```python
from build123d import *

# Parameters (mm, degrees)
SKETCH_1_W          = 20
SKETCH_1_H          = 36
EXTRUDE_1_DEPTH     = 3
SKETCH_2_W          = 33
SKETCH_2_H          = 16
EXTRUDE_2_DEPTH     = 3
EXTRUDE_4_DEPTH     = 6
EXTRUDE_6_DEPTH     = 16
EXTRUDE_7_DEPTH     = 4
SKETCH_13_R         = 1.75
CUT_EXTRUDE_4_DEPTH = 42.261436472
FILLET_3_R          = 2
FILLET_5_R          = 1
SKETCH_14_R         = 1.75
CUT_EXTRUDE_5_DEPTH = 38.098338449
SKETCH_15_R         = 3
CUT_EXTRUDE_6_DEPTH = 1
EXTRUDE_8_DEPTH     = 2


with BuildPart() as part:
    # 草图1 → 凸台-拉伸1 (new body)
    with BuildSketch(Plane(origin=(0, 0, 0), x_dir=(1, 0, 0), z_dir=(0, 1, 0))):
        Rectangle(SKETCH_1_W, SKETCH_1_H)
    extrude(amount=EXTRUDE_1_DEPTH)

    # 草图2 → 凸台-拉伸2 (add)
    with BuildSketch(Plane(origin=(0, 3, 0), x_dir=(1, 0, 0), z_dir=(0, 1, 0))):
        Rectangle(SKETCH_2_W, SKETCH_2_H)
    extrude(amount=-EXTRUDE_2_DEPTH)

    # 草图9 → 凸台-拉伸4 (add, symmetric)
    with BuildSketch(Plane(origin=(0, 0, 0), x_dir=(0, 0, -1), z_dir=(1, 0, 0))):
        Polygon((-11, 3), (-7.89033458, 11.808156288), (8, 3), align=None)
    extrude(amount=EXTRUDE_4_DEPTH, both=True)

    # 草图11 → 凸台-拉伸6 (add)
    with BuildSketch(Plane(origin=(0, 5.687071281, -3.152395087), x_dir=(1, 0, 0), z_dir=(0, 0.8746197071393988, -0.48480962024633173))):
        with BuildLine():
            Line((0.75, -24.683935623), (2.5, -24.683935623))
            Line((2.5, -24.683935623), (2.5, -18.025055397))
            ThreePointArc((2.5, -18.025055397), (0, -6.675749886), (-2.5, -18.025055397))
            Line((-2.5, -18.025055397), (-2.5, -24.683935623))
            Line((-2.5, -24.683935623), (-0.75, -24.683935623))
            Line((-0.75, -24.683935623), (-0.75, -16.503893772))
            ThreePointArc((-0.75, -16.503893772), (0, -8.675749886), (0.75, -16.503893772))
            Line((0.75, -16.503893772), (0.75, -24.683935623))
        make_face()
    extrude(amount=EXTRUDE_6_DEPTH)

    # 草图12 → 凸台-拉伸7 (add, symmetric)
    with BuildSketch(Plane(origin=(0, 0, 0), x_dir=(0, 0, -1), z_dir=(1, 0, 0))):
        Polygon((-4.435586737, 9.893158289), (1.382128706, 20.388594774), (3.435990627, 5.529871706), align=None)
    extrude(amount=EXTRUDE_7_DEPTH, both=True)

    # 草图13 → 切除-拉伸4 (cut, through all)
    with BuildSketch(Plane(origin=(2.5, 0, 0), x_dir=(0, 0, -1), z_dir=(1, 0, 0))):
        with Locations(Location((-9.706952079, 26.535372625, 0), (0, 0, 180))):
            Circle(SKETCH_13_R)
        with Locations(Location((-13.585429041, 19.538414968, 0), (0, 0, 180))):
            Circle(SKETCH_13_R)
    extrude(amount=-CUT_EXTRUDE_4_DEPTH, mode=Mode.SUBTRACT)

    # 圆角3
    fillet_3_edges = [part.edges().sort_by_distance(p)[0] for p in [
        (-1.625, 17.654080736, 18.436661458),
        (1.625, 17.654080736, 18.436661458),
        (-1.625, 31.647996051, 10.679707534),
        (1.625, 31.647996051, 10.679707534),
    ]]
    fillet(fillet_3_edges, radius=FILLET_3_R)

    # 圆角5
    fillet_5_edges = [part.edges().sort_by_distance(p)[0] for p in [
        (16.5, 1.5, 8),
        (-16.5, 1.5, -8),
        (16.5, 1.5, -8),
        (-16.5, 1.5, 8),
        (10, 1.5, 18),
        (-10, 1.5, 18),
        (-10, 1.5, -18),
        (10, 1.5, -18),
    ]]
    fillet(fillet_5_edges, radius=FILLET_5_R)

    # 草图14 → 切除-拉伸5 (cut, through all)
    with BuildSketch(Plane(origin=(0, 3, 0), x_dir=(1, 0, 0), z_dir=(0, 1, 0))):
        with Locations(Location((-6, -14.5, 0), (0, 0, 270))):
            Circle(SKETCH_14_R)
        with Locations(Location((-6, 14.5, 0), (0, 0, 270))):
            Circle(SKETCH_14_R)
        with Locations(Location((6, 14.5, 0), (0, 0, 270))):
            Circle(SKETCH_14_R)
        with Locations(Location((6, -14.5, 0), (0, 0, 270))):
            Circle(SKETCH_14_R)
    extrude(amount=-CUT_EXTRUDE_5_DEPTH, mode=Mode.SUBTRACT)

    # 草图15 → 切除-拉伸6 (cut)
    with BuildSketch(Plane(origin=(0, 3, 0), x_dir=(1, 0, 0), z_dir=(0, 1, 0))):
        with Locations(Location((6, -14.5, 0), (0, 0, 270))):
            Circle(SKETCH_15_R)
        with Locations(Location((-6, -14.5, 0), (0, 0, 270))):
            Circle(SKETCH_15_R)
        with Locations(Location((6, 14.5, 0), (0, 0, 270))):
            Circle(SKETCH_15_R)
        with Locations(Location((-6, 14.5, 0), (0, 0, 270))):
            Circle(SKETCH_15_R)
    extrude(amount=-CUT_EXTRUDE_6_DEPTH, mode=Mode.SUBTRACT)

    # 草图16 → 凸台-拉伸8 (add, symmetric)
    with BuildSketch(Plane(origin=(0, 0, 5.5), x_dir=(-1, 0, 0), z_dir=(0, 0, -1))):
        Polygon((-3.95, 21), (-11.95, 3), (-3.95, 3), align=None)
        Polygon((3.95, 3), (3.95, 21), (11.95, 3), align=None)
    extrude(amount=EXTRUDE_8_DEPTH, both=True)


solid = part.part
```
The model under review builds one solid part; all positions refer to its coordinate system, in mm. A direction names the side the tool comes from. Give positions to 0.01 mm unless a question says otherwise; leave off trailing zeros. Write each loop counter-clockwise with the first axis right and the second up, starting at its lowest first coordinate (ties: lowest second). Pieces come first, ordered by that corner, then holes. Notation, with made-up numbers: M 38,36 L 95,36 A12 ccw 95,44 Z; hole C 36,-35 d3. An arc over 180 degrees is marked long. Answer in a Markdown table with one row per item.
Item 1: Tool access review of faces 1 (the face through (-2.809, 14.212, 12.227)), 2 (the face through (4.2, 2.5, 12.1)), 3 (the face through (10, 1, -12)), 4 (the face through (13, 2, 8)): name each direction out of +Z, -Z, +X, -X, +Y, -Y from which nothing blocks a thin tool from reaching the whole face with its end or side.
Check sheet entries:
| item | result |
|---|---|
| face 1 | +Z, +X, -X |
| face 2 | +Y |
| face 3 | -Z, +X, +Y, -Y |
| face 4 | +Z, +X, +Y, -Y |
Item 2: For line 1 along Z through (x, y) = (4, 2.5); line 2 along X through (y, z) = (0.75, -14.5); line 3 along Y through (x, z) = (-6, -12.5), list the stretches that pass through material, from the lowest coordinate up.
Check sheet entries:
| item | result |
|---|---|
| line 1 | -18 to -16.74, -12.26 to 12.26, 16.74 to 18 |
| line 2 | -10 to -7.75, -4.25 to 4.25, 7.75 to 10 |
| line 3 | 0 to 2 |
Item 3: Add section A-A on y = 29. Give the boundary of the cut face in (x, z), plus the area to 3 significant figures.
Check sheet entries:
| item | result |
|---|---|
| outline | M -2.5,5.9 L -0.75,5.9 L -0.75,12.15 L -2.5,12.15 Z; M 0.75,5.9 L 2.5,5.9 L 2.5,12.15 L 0.75,12.15 Z |
| area | 21.9 mm2 |
Item 4: For P1, Ø0.9, axis at x = 13, y = 1.5, coming from the -Z side; P2, Ø12, axis at x = -9, y = 17, coming from the +Z side; P3, Ø2, axis at y = 26.54, z = 9.71, coming from the -X side; P4, Ø12, axis at y = 5.5, z = 1.5, coming from the +X side, all flat-tipped, find the tip position at first contact; note any pin that passes through.
Check sheet entries:
| item | result |
|---|---|
| P1 | z = -8 |
| P2 | z = 11.91 |
| P3 | through |
| P4 | x = 16.5 |
Item 5: Add section B-B on z = 14.5. State how many separate pieces and enclosed holes the cut face has, plus the area to 3 significant figures.
Check sheet entries:
| item | result |
|---|---|
| separate pieces | 7 |
| enclosed holes | 0 |
| area | 56.1 mm2 |
Item 6: Draft analysis for pull direction X (two halves, no side actions). For faces 5 (the face through (0, 0, 0)), 6 (the face through (4.2, 2.5, -16.9)), 7 (the face through (16.199, 1.479, -7.715)), 8 (the face through (-6, 2, -12.5)), state which applies: +X half, -X half, draft (parallel to the pull), parting line (faces both ways), or undercut.
Check sheet entries:
| item | result |
|---|---|
| face 5 | draft |
| face 6 | undercut |
| face 7 | +X half |
| face 8 | undercut |
